Could you check a few things on this model? Use its own coordinates, in mm. Give positions to 0.01 mm unless a question says otherwise; leave off trailing zeros. Loops run counter-clockwise (first coordinate to the right, second up) from the corner with the lowest first, then second, coordinate; pieces in that order, holes last. Notation, with made-up numbers: M 39.5,50.5 L 80.5,50.5 A37 cw 80.5,89.5 Z; hole C -19.75,-29 d5. An arc over 180 degrees is marked long. Return JSON: item names as keys, results as strings. Group by question number.
1. Please list where these lines run through material, in increasing order: line 1 (X direction, y = 7.5, z = 1.9); line 2 (Y direction, x = 34, z = 0.3); line 3 (Y direction, x = 35, z = 1.9).
2. If we section it at C-C (x = 66.5): Write out the boundary of the cut face in (y, z) (3 decimals), plus the area to 3 significant figures.
3. If we section it at A-A (z = 1.55): Write out the boundary of the cut face in (x, y) (3 decimals), plus the area to 3 significant figures.
4. For pin 1 (1.5 mm diameter, centred on y = 33.5, z = 0.5, fed in from +X) (3 decimals); pin 2 (1 mm diameter, centred on x = 51.5, z = 1, fed in from +Y); pin 3 (1.6 mm diameter, centred on y = -6, z = 1.5, fed in from -X), each with a flat end and sliding along its axis, tell me the tip position at first contact or that it passes through.
5. If we section it at B-B (y = -7.5): Write out the boundary of the cut face in (x, z) (3 decimals).
```python
from build123d import *

# Parameters (mm, degrees)
SKETCH1_W           = 3.175
SKETCH1_H           = 31.75
BOSS_EXTRUDE2_DEPTH = 3.175
SKETCH2_W           = 3.175
SKETCH2_H           = 6.35
BOSS_EXTRUDE3_DEPTH = 3.175


with BuildPart() as part:
    # Sketch1 → Boss-Extrude2 (new body)
    with BuildSketch(Plane.XY):
        Polygon((0, 9.525), (0, -9.525), (98.425, -26.954443488), (98.425, -3.340380987), (98.425, 28.409619013), (98.425, 47.459619012), align=None)
        with Locations((100.0125, 12.534619013)):
            Rectangle(SKETCH1_W, SKETCH1_H)
    extrude(amount=BOSS_EXTRUDE2_DEPTH)

    # Sketch2 → Boss-Extrude3 (add)
    with BuildSketch(Plane.XY.offset(3.175)):
        with Locations((-1.5875, 0)):
            Rectangle(SKETCH2_W, SKETCH2_H)
    extrude(amount=-BOSS_EXTRUDE3_DEPTH)


solid = part.part
```
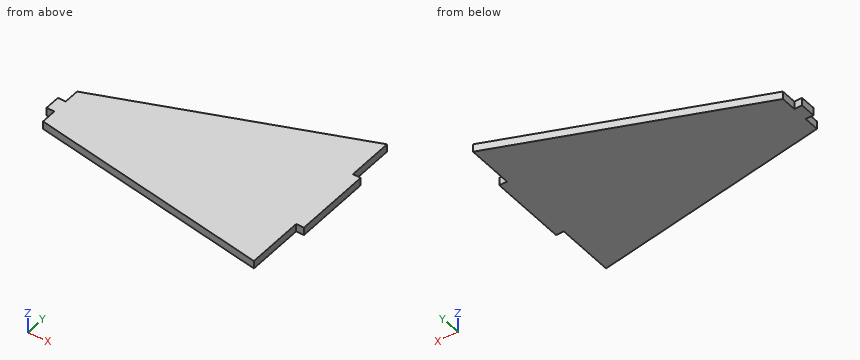
Answer:
{
 "1": {"line 1": "x = 0 to 101.6", "line 2": "y = -15.55 to 22.63", "line 3": "y = -15.72 to 23.01"},
 "2": {"outline": "M -21.301,0 L 35.155,0 L 35.155,3.175 L -21.301,3.175 Z", "area": "179 mm²"},
 "3": {"outline": "M -3.175,-3.175 L 0,-3.175 L 0,-9.525 L 98.425,-26.954 L 98.425,-3.34 L 101.6,-3.34 L 101.6,28.41 L 98.425,28.41 L 98.425,47.46 L 0,9.525 L 0,3.175 L -3.175,3.175 Z", "area": "4,720 mm²"},
 "4": {"pin 1": "stops at x = 98.425", "pin 2": "stops at y = 29.57", "pin 3": "stops at x = 0"},
 "5": {"outline": "M 0,0 L 98.425,0 L 98.425,3.175 L 0,3.175 Z"}
}
